Autodesk Inventor part; units mm, degrees
ref_plane "YZ Plane" through (0, 0, 0) normal (1, 0, 0) x (0, 1, 0)
ref_plane "XZ Plane" through (0, 0, 0) normal (0, 1, 0) x (-1, 0, 0)
ref_plane "XY Plane" through (0, 0, 0) normal (0, 0, 1) x (1, 0, 0)
sketch "Sketch1" plane through (0, 0, 0) normal (0, 1, 0) x (-1, 0, 0)
  line L0 (0, 0) -> (-23, 0)
  line L1 (-23, 0) -> (-23, -20)
  line L2 (-23, -20) -> (0, -20)
  line L3 (0, -20) -> (0, 0)
  line L4 (-13, -20) -> (-13, 0)
  point P0 (-18, -10)
  point P1 (-23, -10)
  point P2 (-6.5, -10)
  point P3 (0, -10)
  dimension "d0" = 20
  dimension "d5" = 13
  dimension "d7" = 5
  dimension "d8" = 5
  dimension "d25" = 6.5
extrude "Extrusion1" add sketch "Sketch1" against normal blind 6
hole "Hole2" at (6.5, 0, -10) direction (0, -1, 0) diameter 3.4036 end through all
sketch "Sketch3" plane through (0, -6, 0) normal (0, -1, 0) x (1, 0, 0)
  circle A0 centre (6.5, -10) radius 1.7018 construction
  line L0 (9.6754, -10) -> (8.0877, -12.75)
  line L1 (8.0877, -12.75) -> (4.9123, -12.75)
  line L2 (4.9123, -12.75) -> (3.3246, -10)
  line L3 (3.3246, -10) -> (4.9123, -7.25)
  line L4 (4.9123, -7.25) -> (8.0877, -7.25)
  line L5 (8.0877, -7.25) -> (9.6754, -10)
  dimension "d33" = 5.5
extrude "Extrusion4" cut sketch "Sketch3" against normal blind 2.2
extrude "Extrusion2" add sketch "Sketch1" along normal blind 6 contours L4 L2 L1 L0
sketch "Sketch2" plane through (0, 6, 0) normal (0, 1, 0) x (1, 0, 0)
  point P0 (18, 10)
hole "Hole1" at (18, 6, -10) direction (0, -1, 0) diameter 3.4036 end through all counterbore diameter 6.5024 counterbore depth 2.9972
chamfer "Chamfer1" distance 0.6 angle 45 18 edges at (6.5, 0, -20) (13, 3, -20) (18, 6, -20) (23, 6, -10) (18, 6, 0) (13, 3, 0) (6.5, 0, 0) (0, -3, 0) (23, 0, 0) (23, 0, -20) (11.5, -6, -20) (23, -6, -10) (11.5, -6, 0) (0, -6, -10) (0, -3, -20) (18, 6, -13.2512) (0, 0, -10) (13, 6, -10)
Can you work these out from the model? Positions are in its coordinate system, mm. A direction names the side the tool comes from. Round coordinates to 2 decimals unless told otherwise and drop trailing zeros. Write each loop counter-clockwise with the first axis right and the second up, starting at its lowest first coordinate (ties: lowest second). Pieces come first, ordered by that corner, then holes. Notation, with made-up numbers: M -17.5,74 L -3.5,74 A6 ccw -3.5,84 Z; hole C -4,64 d8. An arc over 180 degrees is marked long. Use a Markdown table: item, result.
Item 1: If I drill on line 1 along X through (y, z) = (-2.25, -10); line 2 along Z through (x, y) = (6.5, -1.7); line 3 along X through (y, z) = (-4.5, -10.25), over which ranges is the centre line in solid material (lowest first)? Write a range as [from, to].
Found:
| item | result |
|---|---|
| line 1 | x = [0, 4.8], [8.2, 16.3], [19.7, 23] |
| line 2 | z = [-20, -11.7], [-8.3, 0] |
| line 3 | x = [0, 3.47], [9.53, 16.32], [19.68, 23] |
Item 2: We'd pull the mould along X, two halves only. Please class faces 1 (the face through (8.87, -4.915, -8.606)), 2 (the face through (23, 0, -10)), 3 (the face through (22, 6, -9.9)): released by +X, released by -X, zero draft, split by the parting line, or undercut.
Found:
| item | result |
|---|---|
| face 1 | undercut |
| face 2 | released by +X |
| face 3 | zero draft |
Item 3: I want a section at C-C (z = -16). List the corners of the cut face in (x, y) for me, and give its area (3 significant figures).
Found:
| item | result |
|---|---|
| outline | M 0,-5.4 L 0.6,-6 L 22.4,-6 L 23,-5.4 L 23,5.4 L 22.4,6 L 13.6,6 L 13,5.4 L 13,0 L 0.6,0 L 0,-0.6 Z |
| area | 197 mm2 |
Item 4: I want a section at B-B (y = -2.75). List the corners of the cut face in (x, z) for me.
Found:
| item | result |
|---|---|
| outline | M 0,-19.4 L 0.6,-20 L 22.4,-20 L 23,-19.4 L 23,-0.6 L 22.4,0 L 0.6,0 L 0,-0.6 Z; hole C 6.5,-10 d3.4; hole C 18,-10 d3.4 |
Item 5: I want a section at A-A (x = 18). List the corners of the cut face in (y, z) for me.
Found:
| item | result |
|---|---|
| outline | M -6,-19.4 L -5.4,-20 L 5.4,-20 L 6,-19.4 L 6,-13.85 L 5.4,-13.25 L 3,-13.25 L 3,-11.7 L -6,-11.7 Z; M -6,-8.3 L 3,-8.3 L 3,-6.75 L 5.4,-6.75 L 6,-6.15 L 6,-0.6 L 5.4,0 L -5.4,0 L -6,-0.6 Z |
Item 6: For pin 1 Ø8.5 at (x, z) = (18, -10) entering from -Y; pin 2 Ø4 at (x, z) = (6.5, -10) entering from +Y; pin 3 Ø4.5 at (y, z) = (2.5, -6) entering from -X; pin 4 Ø1.6 at (x, z) = (6, -10) entering from -Y, each with a flat end and sliding along its axis, tell me the tip position at first contact or that it passes through.
Found:
| item | result |
|---|---|
| pin 1 | stops at y = -6 |
| pin 2 | stops at y = 0 |
| pin 3 | stops at x = 13 |
| pin 4 | passes through |
Item 7: Which directions (+Z, -Z, +X, -X, +Y, -Y) give clear straight access to the entire face, cutting with the end or side of a thin tool? Please do faces 4 (the face through (6, -5, -7.25)), 5 (the face through (13, 3, -10)), 6 (the face through (14, -1, -20)), 7 (the face through (17.86, 4.18, -13.25)).
Found:
| item | result |
|---|---|
| face 4 | -Y |
| face 5 | +Z, -Z, -X, +Y |
| face 6 | -Z, +X, -X, +Y, -Y |
| face 7 | +Y |
Item 8: I want a section at D-D (y = 1.5). List the corners of the cut face in (x, z) for me.
Found:
| item | result |
|---|---|
| outline | M 13,-19.4 L 13.6,-20 L 22.4,-20 L 23,-19.4 L 23,-0.6 L 22.4,0 L 13.6,0 L 13,-0.6 Z; hole C 18,-10 d3.4 |
